```python
from build123d import *

# Parameters (mm, degrees)
SKETCH_1_W                = 11
SKETCH_1_H                = 2
SKETCH_2_R                = 10
EXTRUDE_1_DEPTH           = 14.5
HOLE_WIZARD_3_0_3_1_D     = 3
HOLE_WIZARD_3_0_3_1_DEPTH = 6
HOLE_WIZARD_10_0_10_1_D   = 10


with BuildPart() as part:
    # 草图1 → 旋转1 (revolve)
    with BuildSketch(Plane.XY, mode=Mode.PRIVATE) as revolve_1_sk:
        with Locations((5.5, 1)):
            Rectangle(SKETCH_1_W, SKETCH_1_H)
    revolve(revolve_1_sk.sketch.rotate(Axis((0, 2, 0), (0, -1, 0)), 270), axis=Axis((0, 2, 0), (0, -1, 0)))

    # 草图2 → 凸台-拉伸1 (add)
    with BuildSketch(Plane(origin=(0, 2, 0), x_dir=(-1, 0, 0), z_dir=(0, 1, 0))):
        with Locations(Location((0, 0, 0), (0, 0, 270))):
            Circle(SKETCH_2_R)
    extrude(amount=EXTRUDE_1_DEPTH)

    # Ø3.0 (3) 直径孔1
    with Locations(Plane(origin=(0, 16.5, 0), x_dir=(1, 0, 0), z_dir=(0, 1, 0))):
        with Locations((5.303300859, 5.303300859), (5.303300859, -5.303300859), (-5.303300859, -5.303300859), (-5.303300859, 5.303300859)):
            Hole(HOLE_WIZARD_3_0_3_1_D / 2, depth=HOLE_WIZARD_3_0_3_1_DEPTH)

    # Ø10.0 (10) 直径孔1 (through all)
    with Locations(Plane(origin=(0, 0, 0), x_dir=(-1, 0, 0), z_dir=(0, -1, 0))):
        with Locations((0, 0)):
            Hole(HOLE_WIZARD_10_0_10_1_D / 2)


solid = part.part
```
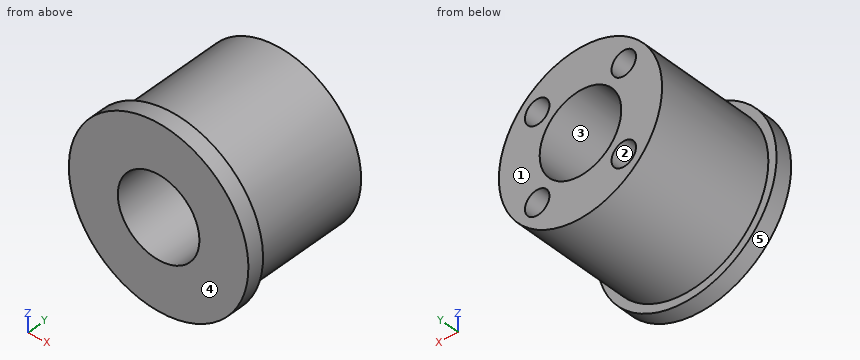
Input: part model. Units: mm. Frame: model coordinates. Face numbers are marked on the shaded views. A direction names the side the tool comes from. Give positions to 0.01 mm unless a question says otherwise; leave off trailing zeros. Order: outer loops, then holes, each group sorted by start corner. A loop starts at its lowest first (then second) coordinate and runs counter-clockwise, first axis right, second up. Notation, with made-up numbers: (66, -34) - (106, -34) arc R19 ccw to (106, 3) - close; hole circle Ø1 at (-35.5, 68.5). An arc over 180 degrees is marked (long way). Put each result on its own line as item: value.
Item 1: Access query for the marked faces 1 and 2. Directions: +Z, -Z, +X, -X, +Y, -Y. A direction counts if a zero-diameter tool reaches every point of the face in a straight line with its end or side. Return the directions, or none.
Found:
face 1: +Z, -Z, +X, -X, +Y
face 2: +Y
Item 2: Contact query for flat-ended pins moving along their axis: pin 1 (1 mm diameter, centred on x = -6.5, z = -6, fed in from +Y); pin 2 (3 mm diameter, centred on x = -8, y = 6.5, fed in from +Z); pin 3 (0.9 mm diameter, centred on x = 5, z = 5.5, fed in from +Y); pin 4 (2 mm diameter, centred on x = -3.5, y = 9.5, fed in from +Z). Output: stop coordinate, or through.
Found:
pin 1: stops at y = 16.5
pin 2: stops at z = 7.6
pin 3: stops at y = 10.5
pin 4: stops at z = 9.68
Item 3: Draft query along Z for the marked faces 3, 4 and 5. Return one class per face: +Z half, -Z half, draft (parallel to the pull), parting line (faces both ways), or undercut.
Found:
face 3: undercut
face 4: draft
face 5: parting line
Item 4: Section query B-B, the plane x = 0. Return loops of the section in (y, z).
Found:
outline: (0, -11) - (2, -11) - (2, -10) - (16.5, -10) - (16.5, -5) - (0, -5) - close; (0, 5) - (16.5, 5) - (16.5, 10) - (2, 10) - (2, 11) - (0, 11) - close
Item 5: Section query A-A, the plane z = 0. Return loops of the section in (x, y).
Found:
outline: (-11, 0) - (-5, 0) - (-5, 16.5) - (-10, 16.5) - (-10, 2) - (-11, 2) - close; (5, 0) - (11, 0) - (11, 2) - (10, 2) - (10, 16.5) - (5, 16.5) - close
Item 6: Section query D-D, the plane y = 15.5. Return loops of the section in (x, z).
Found:
outline: circle Ø20 at (0, 0); hole circle Ø3 at (-5.3, -5.3); hole circle Ø3 at (-5.3, 5.3); hole circle Ø10 at (0, 0); hole circle Ø3 at (5.3, -5.3); hole circle Ø3 at (5.3, 5.3)
Item 7: Ray query, L1, parallel to Z at x = -5.25, y = 15.5; L2, parallel to Z at x = -1, y = 7; L3, parallel to Z at x = 1.5, y = 13.25. Return the intervals inside material, ascending. Write a range as from..to.
Found:
L1: z = -8.51..-6.8, -3.8..3.8, 6.8..8.51
L2: z = -9.95..-4.9, 4.9..9.95
L3: z = -9.89..-4.77, 4.77..9.89
Item 8: Section query C-C, the plane z = -9. Return loops of the section in (x, y).
Found:
outline: (-6.32, 0) - (6.32, 0) - (6.32, 2) - (4.36, 2) - (4.36, 16.5) - (-4.36, 16.5) - (-4.36, 2) - (-6.32, 2) - close
